Part model, mm, in its own coordinate system. Face numbers are marked on the shaded views. A direction names the side the tool comes from. Round coordinates to 2 decimals unless told otherwise and drop trailing zeros. Loops run counter-clockwise (first coordinate to the right, second up) from the corner with the lowest first, then second, coordinate; pieces in that order, holes last. Notation, with made-up numbers: (-6, 67) - (34, 67) arc R15 cw to (34, 89) - close; hole circle Ø7 at (21.5, 69). An arc over 180 degrees is marked (long way). Write each question's results on one line, items separated by ' | '. Start each with the question number.
(1) Flat gauge pins, fed straight in: P1, Ø5.5, axis at x = -14.25, z = 0, coming from the -Y side; P2, Ø3, axis at x = -15, z = -27, coming from the +Y side; P3, Ø4, axis at x = 30, z = -20, coming from the -Y side; P4, Ø3, axis at y = 95.7, z = 48.375, coming from the +X side. Where does each tip first touch, or does it go through?
(2) Mould opens along Z. For the marked faces 3, 4, 5 and 6 say: released by +Z, released by -Z, zero draft, split by the parting line, or undercut.
(3) Cut at D-D, the plane z = -7. List the corners of the cut face in (x, y).
(4) Cut at B-B, the plane y = 34.5. List the corners of the cut face in (x, z).
(5) Cut at A-A, the plane x = -14.25. List the corners of the cut face in (y, z), then the cut area to 3 significant figures.
(6) Tool access for the marked faces 1 and 2: list every direction of +Z, -Z, +X, -X, +Y, -Y with a clear straight run to the whole face (end or side of a thin tool).
(7) Cut at C-C, the plane z = -20. List the corners of the cut face in (x, y), then the cut area to 3 significant figures.
(8) Drill centre lines: L1, parallel to Z at x = -19, y = 79; L2, parallel to X at y = 72, z = 15.5; L3, parallel to X at y = 1.15, z = 0. Where is each one in solid material? Low to high.
from build123d import *

# Parameters (mm, degrees)
SKETCH1_W           = 100
SKETCH1_H           = 100
BOSS_EXTRUDE1_DEPTH = 90
SKETCH2_W           = 96
SKETCH2_H           = 93
CUT_EXTRUDE1_DEPTH  = 88
CUT_EXTRUDE2_REACH  = 4
SKETCH3_R           = 3
SKETCH3_R_2         = 1.75
CHAMFER1_SIZE       = 0.8
SKETCH4_W           = 10
SKETCH4_H           = 5
BOSS_EXTRUDE2_DEPTH = 7.7
SKETCH5_R           = 1.25
CUT_EXTRUDE3_DEPTH  = 91
FILLET1_R           = 3
FILLET2_R           = 4
FILLET3_R           = 1


with BuildPart() as part:
    # Sketch1 → Boss-Extrude1 (new body)
    with BuildSketch(Plane(origin=(0, 0, 0), x_dir=(1, 0, 0), z_dir=(0, 1, 0))):
        Rectangle(SKETCH1_W, SKETCH1_H)
    extrude(amount=BOSS_EXTRUDE1_DEPTH)

    # Sketch2 → Cut-Extrude1 (cut)
    with BuildSketch(Plane(origin=(0, 90, 0), x_dir=(1, 0, 0), z_dir=(0, 1, 0))):
        with Locations((0, 1.5)):
            Rectangle(SKETCH2_W, SKETCH2_H)
    extrude(amount=-CUT_EXTRUDE1_DEPTH, mode=Mode.SUBTRACT)

    # Sketch3 → Cut-Extrude2 (cut, up to next)
    with BuildSketch(Plane(origin=(0, 2, 0), x_dir=(1, 0, 0), z_dir=(0, 1, 0)), mode=Mode.PRIVATE) as cut_extrude2_sk1:
        with Locations((-14.25, 0)):
            Circle(SKETCH3_R)
    cut_extrude2_tool1 = extrude(cut_extrude2_sk1.sketch, amount=-CUT_EXTRUDE2_REACH, mode=Mode.PRIVATE) & part.part
    add(cut_extrude2_tool1.solids().sort_by_distance((-14.25, 2, 0))[0], mode=Mode.SUBTRACT)
    # Sketch3 → Cut-Extrude2 (cut, up to next)
    with BuildSketch(Plane(origin=(0, 2, 0), x_dir=(1, 0, 0), z_dir=(0, 1, 0)), mode=Mode.PRIVATE) as cut_extrude2_sk2:
        with Locations((-30, 20)):
            Circle(SKETCH3_R_2)
    cut_extrude2_tool2 = extrude(cut_extrude2_sk2.sketch, amount=-CUT_EXTRUDE2_REACH, mode=Mode.PRIVATE) & part.part
    add(cut_extrude2_tool2.solids().sort_by_distance((-30, 2, -20))[0], mode=Mode.SUBTRACT)
    # Sketch3 → Cut-Extrude2 (cut, up to next)
    with BuildSketch(Plane(origin=(0, 2, 0), x_dir=(1, 0, 0), z_dir=(0, 1, 0)), mode=Mode.PRIVATE) as cut_extrude2_sk3:
        with Locations((-30, -20)):
            Circle(SKETCH3_R_2)
    cut_extrude2_tool3 = extrude(cut_extrude2_sk3.sketch, amount=-CUT_EXTRUDE2_REACH, mode=Mode.PRIVATE) & part.part
    add(cut_extrude2_tool3.solids().sort_by_distance((-30, 2, 20))[0], mode=Mode.SUBTRACT)
    # Sketch3 → Cut-Extrude2 (cut, up to next)
    with BuildSketch(Plane(origin=(0, 2, 0), x_dir=(1, 0, 0), z_dir=(0, 1, 0)), mode=Mode.PRIVATE) as cut_extrude2_sk4:
        with Locations((30, -20)):
            Circle(SKETCH3_R_2)
    cut_extrude2_tool4 = extrude(cut_extrude2_sk4.sketch, amount=-CUT_EXTRUDE2_REACH, mode=Mode.PRIVATE) & part.part
    add(cut_extrude2_tool4.solids().sort_by_distance((30, 2, 20))[0], mode=Mode.SUBTRACT)
    # Sketch3 → Cut-Extrude2 (cut, up to next)
    with BuildSketch(Plane(origin=(0, 2, 0), x_dir=(1, 0, 0), z_dir=(0, 1, 0)), mode=Mode.PRIVATE) as cut_extrude2_sk5:
        with Locations((30, 20)):
            Circle(SKETCH3_R_2)
    cut_extrude2_tool5 = extrude(cut_extrude2_sk5.sketch, amount=-CUT_EXTRUDE2_REACH, mode=Mode.PRIVATE) & part.part
    add(cut_extrude2_tool5.solids().sort_by_distance((30, 2, -20))[0], mode=Mode.SUBTRACT)
    # Sketch3 → Cut-Extrude2 (cut, up to next)
    with BuildSketch(Plane(origin=(0, 2, 0), x_dir=(1, 0, 0), z_dir=(0, 1, 0)), mode=Mode.PRIVATE) as cut_extrude2_sk6:
        with BuildLine():
            Line((0, 1.25), (22, 1.25))
            ThreePointArc((22, 1.25), (23.25, 0), (22, -1.25))
            Line((22, -1.25), (0, -1.25))
            ThreePointArc((0, -1.25), (-1.25, 0), (0, 1.25))
        make_face()
    cut_extrude2_tool6 = extrude(cut_extrude2_sk6.sketch, amount=-CUT_EXTRUDE2_REACH, mode=Mode.PRIVATE) & part.part
    add(cut_extrude2_tool6.solids().sort_by_distance((11, 2, 0))[0], mode=Mode.SUBTRACT)

    # Chamfer1
    chamfer1_edges = [part.edges().sort_by_distance(p)[0] for p in [
        (-31.75, 0, -20),
        (-31.75, 0, 20),
        (28.25, 0, 20),
        (28.25, 0, -20),
    ]]
    chamfer(chamfer1_edges, length=CHAMFER1_SIZE)

    # Sketch4 → Boss-Extrude2 (add)
    with BuildSketch(Plane(origin=(0, 90, 0), x_dir=(1, 0, 0), z_dir=(0, 1, 0))):
        with Locations((-35, -47.5)):
            Rectangle(SKETCH4_W, SKETCH4_H)
        with Locations((35, -47.5)):
            Rectangle(SKETCH4_W, SKETCH4_H)
    extrude(amount=BOSS_EXTRUDE2_DEPTH)

    # Sketch5 → Cut-Extrude3 (cut, through all)
    with BuildSketch(Plane.ZY.offset(40)):
        with Locations((48.375, 95.7)):
            Circle(SKETCH5_R)
    extrude(amount=-CUT_EXTRUDE3_DEPTH, mode=Mode.SUBTRACT)

    # Fillet1
    fillet1_edges = [part.edges().sort_by_distance(p)[0] for p in [
        (-48, 2, -1.5),
        (-48, 46, 45),
        (0, 2, 45),
        (48, 46, 45),
        (48, 2, -1.5),
        (48, 46, -48),
        (0, 2, -48),
        (-48, 46, -48),
    ]]
    fillet(fillet1_edges, radius=FILLET1_R)

    # Fillet2
    fillet2_edges = [part.edges().sort_by_distance(p)[0] for p in [
        (0, 0, 50),
        (-50, 0, 0),
        (0, 0, -50),
        (50, 0, 0),
        (50, 45, 50),
        (-50, 45, 50),
        (-50, 45, -50),
        (50, 45, -50),
    ]]
    fillet(fillet2_edges, radius=FILLET2_R)

    # Fillet3
    fillet3_edges = [part.edges().sort_by_distance(p)[0] for p in [
        (-35, 97.7, 45),
        (35, 97.7, 45),
    ]]
    fillet(fillet3_edges, radius=FILLET3_R)


solid = part.part
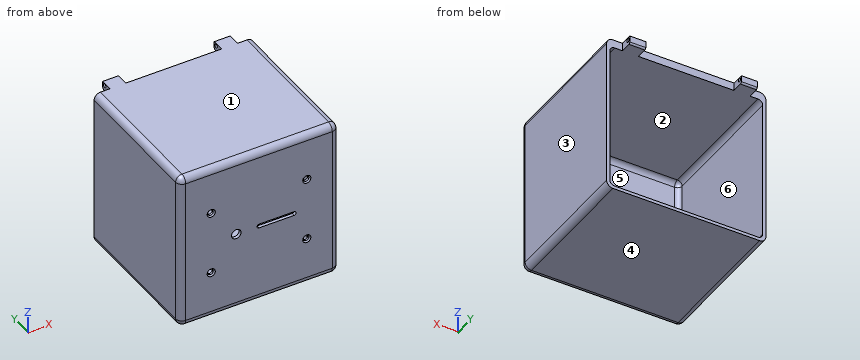
A:
1) P1: through | P2: y = 2 | P3: y = 0.55 | P4: x = 40
2) face 3: zero draft | face 4: released by -Z | face 5: undercut | face 6: undercut
3) outline: (-50, 4) arc R4 ccw to (-46, 0) - (46, 0) arc R4 ccw to (50, 4) - (50, 90) - (48, 90) - (48, 5) arc R3 cw to (45, 2) - (-45, 2) arc R3 cw to (-48, 5) - (-48, 90) - (-50, 90) - close
4) outline: (-50, -46) arc R4 ccw to (-46, -50) - (46, -50) arc R4 ccw to (50, -46) - (50, 46) arc R4 ccw to (46, 50) - (-46, 50) arc R4 ccw to (-50, 46) - close; hole (-48, -45) arc R3 ccw to (-45, -48) - (45, -48) arc R3 ccw to (48, -45) - (48, 42) arc R3 ccw to (45, 45) - (-45, 45) arc R3 ccw to (-48, 42) - close
5) outline: (0, -46) arc R4 ccw to (4, -50) - (90, -50) - (90, -48) - (5, -48) arc R3 cw to (2, -45) - (2, -3) - (0, -3) - close; (0, 3) - (2, 3) - (2, 42) arc R3 cw to (5, 45) - (90, 45) - (90, 50) - (4, 50) arc R4 ccw to (0, 46) - close | area: 801 mm2
6) face 1: +Z, +X, -X, +Y, -Y | face 2: +Y
7) outline: (-50, 4) arc R4 ccw to (-46, 0) - (-32.55, 0) - (-31.75, 0.8) - (-31.75, 2) - (-45, 2) arc R3 cw to (-48, 5) - (-48, 90) - (-50, 90) - close; (-28.25, 0.8) - (-27.45, 0) - (27.45, 0) - (28.25, 0.8) - (28.25, 2) - (-28.25, 2) - close; (31.75, 0.8) - (32.55, 0) - (46, 0) arc R4 ccw to (50, 4) - (50, 90) - (48, 90) - (48, 5) arc R3 cw to (45, 2) - (31.75, 2) - close | area: 534 mm2
8) L1: -50 to -48, 45 to 50 | L2: -50 to -48, 48 to 50 | L3: -48.81 to -17.25, -11.25 to -1.25, 23.25 to 48.81
